Autodesk Inventor part; units mm, degrees
ref_plane "YZ Plane" through (0, 0, 0) normal (1, 0, 0) x (0, 1, 0)
ref_plane "XZ Plane" through (0, 0, 0) normal (0, 1, 0) x (-1, 0, 0)
ref_plane "XY Plane" through (0, 0, 0) normal (0, 0, 1) x (1, 0, 0)
sketch "Sketch1" plane through (0, 0, 0) normal (0, 1, 0) x (-1, 0, 0)
  line L0 (15, 20.25) -> (-15, 20.25)
  line L1 (-15, 20.25) -> (-15, -20.25)
  line L2 (-15, -20.25) -> (15, -20.25)
  line L3 (15, -20.25) -> (15, 20.25)
  line L4 (15, 20.25) -> (-15, -20.25) construction
  line L5 (-15, 20.25) -> (15, -20.25) construction
  point P0 (0, 0)
  dimension "d0" = 30
  dimension "d1" = 40.5
extrude "Plate1" add sketch "Sketch1" along normal blind 1.5
sketch "Sketch2" plane through (15, 0, 21.75) normal (0, 0, -1) x (-1, 0, 0)
  line L0 (30, 0) -> (0, 0)
  line L1 (0, 0) -> (0, 30)
  line L2 (0, 30) -> (30, 30)
  line L3 (30, 30) -> (30, 0)
edge flange "Flange1" height 30 angle 90 thickness 1.5 bend radius 0.31 thickness toward (0, 0, -1) relief tear relief width 1.5 relief depth 0.75 corner gap 0.31 corner form 0 edges at (0, 1.5, 20.25) (0, 1.5, -20.25) wall of the first edge with corners at (-15, 0, 21.75) (15, 0, 21.75) (15, 30, 21.75) (-15, 30, 21.75)
bend "Bend1"
corner "Corner1"
sketch "Sketch3" plane through (-15, 30, 21.75) normal (0, 0, 1) x (1, 0, 0)
  circle A0 centre (22.525, -21) radius 0.7835
  circle A1 centre (22.525, -5.9) radius 0.7835
  circle A2 centre (7.475, -21) radius 0.7835
  circle A3 centre (7.475, -5.9) radius 0.7835
  ellipse E0 centre (22.952, 14.482) end of major axis (23.818, 15.348) minor radius 1 (24.07, 14.7056) -> (23.1756, 15.6) ccw
  line L0 (6.8244, 15.6) -> (23.1756, 15.6)
  ellipse E1 centre (7.048, 14.482) end of major axis (6.182, 15.348) minor radius 1 (6.8244, 15.6) -> (5.93, 14.7056) ccw
  line L1 (5.93, -21.6056) -> (5.93, 14.7056)
  ellipse E2 centre (7.048, -21.382) end of major axis (6.182, -22.248) minor radius 1 (5.93, -21.6056) -> (6.8244, -22.5) ccw
  line L2 (23.1756, -22.5) -> (6.8244, -22.5)
  ellipse E3 centre (22.952, -21.382) end of major axis (23.818, -22.248) minor radius 1 (23.1756, -22.5) -> (24.07, -21.6056) ccw
  line L3 (24.07, 14.7056) -> (24.07, -21.6056)
  circle A4 centre (7.475, -21) radius 0.7835
  circle A5 centre (22.525, -21) radius 0.7835
  circle A6 centre (7.475, -5.9) radius 0.7835
  circle A7 centre (22.525, -5.9) radius 0.7835
  circle A8 centre (7.475, 14.1) radius 0.7835
  circle A9 centre (22.525, 14.1) radius 0.7835
  circle A10 centre (15, 6.6) radius 6.4
  point P0 (15, -30)
hole "Hole1" at (7.525, 24.1, 21.75) at (7.525, 9, 21.75) at (-7.525, 9, 21.75) at (-7.525, 24.1, 21.75) direction (0, 0, -1) diameter 2.1 depth 1.5
sketch "Sketch4" plane through (15, 30, -21.75) normal (0, 0, -1) x (-1, 0, 0)
  circle A0 centre (15, -20.82) radius 0.7835
  circle A1 centre (8, -13.52) radius 0.7835
  circle A2 centre (22, -13.52) radius 0.7835
  circle A3 centre (7, -0.3) radius 0.7835
  circle A4 centre (23, -0.3) radius 0.7835
  line L0 (21.07, -22.22) -> (8.93, -22.22)
  line L1 (21.07, -22.22) -> (21.07, -21.5)
  arc A5 (23.07, -19.5) -> (21.07, -21.5) centre (23.07, -21.5) ccw
  line L2 (23.07, -19.5) -> (23.79, -19.5)
  line L3 (23.79, 12.6) -> (23.79, -19.5)
  line L4 (23.79, 12.6) -> (23.07, 12.6)
  arc A6 (21.07, 14.6) -> (23.07, 12.6) centre (23.07, 14.6) ccw
  line L5 (21.07, 14.6) -> (21.07, 15.32)
  line L6 (8.93, 15.32) -> (21.07, 15.32)
  line L7 (8.93, 15.32) -> (8.93, 14.6)
  arc A7 (6.93, 12.6) -> (8.93, 14.6) centre (6.93, 14.6) ccw
  line L8 (6.93, 12.6) -> (6.21, 12.6)
  line L9 (6.21, -19.5) -> (6.21, 12.6)
  line L10 (6.21, -19.5) -> (6.93, -19.5)
  arc A8 (8.93, -21.5) -> (6.93, -19.5) centre (6.93, -21.5) ccw
  line L11 (8.93, -21.5) -> (8.93, -22.22)
  circle A9 centre (15, 6.6) radius 6.4
  point P0 (15, -30)
hole "Hole2" at (-7, 16.48, -21.75) at (7, 16.48, -21.75) at (0, 9.18, -21.75) direction (0, 0, 1) diameter 2.1 depth 1.5
equation "\"d18\" = Thickness"
equation "\"d25\" = Thickness"
equation "\"d2\" = Thickness"
equation "\"d3\" = BendReliefWidth"
equation "\"d4\" = BendReliefDepth"
equation "\"d5\" = MinimumRemnant"
equation "\"d6\" = TransitionRadius"
equation "\"d9\" = BendRadius"
equation "\"d10\" = CornerReliefSize"
equation "\"d11\" = GapSize"
equation "\"d12\" = JacobiRadiusSize"
equation "\"BendReliefWidth\" = Thickness"
equation "\"BendReliefDepth\" = 0.5 * Thickness"
equation "\"CornerReliefSize\" = 4 * Thickness"
equation "\"MinimumRemnant\" = 2 * Thickness"
equation "\"TransitionRadius\" = BendRadius"
equation "\"JacobiRadiusSize\" = BendRadius"
equation "\"GapSize\" = Thickness"
properties part number "HWFrame" material "Aluminum 6061-AHC"
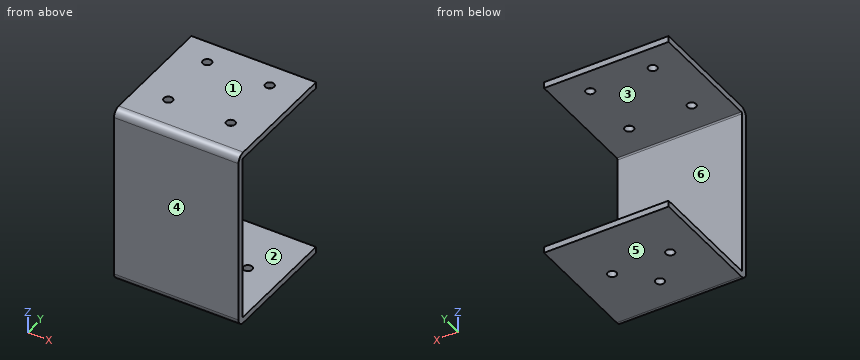
CAD build for the part. Positions are in the model's coordinates, mm. Face numbers are marked on the shaded views. A direction names the side the tool comes from. Round coordinates to 2 decimals unless told otherwise and drop trailing zeros. Write each loop counter-clockwise with the first axis right and the second up, starting at its lowest first coordinate (ties: lowest second). Pieces come first, ordered by that corner, then holes. Notation, with made-up numbers: (80.5, -15.5) - (130.5, -15.5) arc R20 cw to (130.5, 10.5) - close; hole circle Ø4 at (89.5, 49). An arc over 180 degrees is marked (long way). Write item = value, one per line. Start each with the question number.
Q1. Band-saw the part on A-A (y = 6.75). Give the cut face in (x, z), then the cut area to 3 significant figures.
Q2. Band-saw the part on D-D (z = -7.5). Give the cut face in (x, y).
Q3. Drop flat-ended pins along their axis: pin 1 (8 mm diameter, centred on y = 7.5, z = -14.5, fed in from +X); pin 2 (5 mm diameter, centred on x = 6.5, z = 2.5, fed in from +Y); pin 3 (1.9 mm diameter, centred on x = 7, y = 16.48, fed in from -Z); pin 4 (6 mm diameter, centred on x = -2, z = -16.5, fed in from -Y). Give the stop position or say it passes through.
Q4. Which spindle directions (+Z, -Z, +X, -X, +Y, -Y) get a long thin tool onto all of the face, cutting with end or side? Do the marked faces 5 and 6. Say none if no direction does.
Q5. Mould opens along Z. For the marked faces 1, 2, 3 and 4 say: pulls with the +Z half, pulls with the -Z half, needs draft (parallel to the pull), parting line crosses it, or undercut.
Q6. Probe L1, parallel to X at y = 16.48, z = -21.35; L2, parallel to X at y = 9, z = 20.7 (3 decimals); L3, parallel to Z at x = 11.25, y = 28.5. List the from-to ranges inside material, lowest first. Write a range as from..to.
Q7. Band-saw the part on B-B (x = 9.5). Give the cut face in (y, z).
Q8. Band-saw the part on C-C (y = 16.48). Give the cut face in (x, z).
Answers below:
q1.outline = (-15, -21.75) - (15, -21.75) - (15, -20.25) - (-15, -20.25) - close; (-15, 20.25) - (15, 20.25) - (15, 21.75) - (-15, 21.75) - close
q1.area = 90.0 mm2
q2.outline = (-15, 0) - (15, 0) - (15, 1.5) - (-15, 1.5) - close
q3.pin_1 = through
q3.pin_2 = 1.5
q3.pin_3 = 20.25
q3.pin_4 = 0
q4.face_5 = -Z, +X, -X, +Y, -Y
q4.face_6 = +X, -X, +Y
q5.face_1 = pulls with the +Z half
q5.face_2 = undercut
q5.face_3 = undercut
q5.face_4 = needs draft
q6.L1 = -15..-8.05, -5.95..5.95, 8.05..15
q6.L2 = -15..-8.575, -6.475..6.475, 8.575..15
q6.L3 = -21.75..-20.25, 20.25..21.75
q7.outline = (0, -19.94) arc R1.81 ccw to (1.81, -21.75) - (30, -21.75) - (30, -20.25) - (1.81, -20.25) arc R0.31 cw to (1.5, -19.94) - (1.5, 19.94) arc R0.31 cw to (1.81, 20.25) - (30, 20.25) - (30, 21.75) - (1.81, 21.75) arc R1.81 ccw to (0, 19.94) - close
q8.outline = (-15, -21.75) - (-8.05, -21.75) - (-8.05, -20.25) - (-15, -20.25) - close; (-15, 20.25) - (15, 20.25) - (15, 21.75) - (-15, 21.75) - close; (-5.95, -21.75) - (5.95, -21.75) - (5.95, -20.25) - (-5.95, -20.25) - close; (8.05, -21.75) - (15, -21.75) - (15, -20.25) - (8.05, -20.25) - close
